Can you work these out from the model? Positions are in its coordinate system, mm. A direction names the side the tool comes from. Give positions to 0.01 mm unless a question says otherwise; leave off trailing zeros. Loops run counter-clockwise (first coordinate to the right, second up) from the corner with the lowest first, then second, coordinate; pieces in that order, holes last. Notation, with made-up numbers: (-19.5, 26) -> (-2.5, 26) arc R27 cw to (-2.5, 43) -> close; hole circle Ø11 at (56, 64). An arc over 180 degrees is marked (long way). Return JSON: item names as keys, results as strings. Group by question number.
Q1. Which directions (+Z, -Z, +X, -X, +Y, -Y) give clear straight access to the entire face, cutting with the end or side of a thin tool? Please do faces 4 (the flat face through (-1.2, -20, -8)), 5 (the cylindrical face through (0.112, -9.86, -5.074)), 6 (the flat face through (0, -36, 0)).
Q2. Suppose I cut it at A-A, the plane z = -8. Please give me the cut outline in (x, y), and give its area (3 significant figures).
Q3. Thinking about a two-plate mould opening in Z: for faces 1 (the flat face through (-4, -20, -8.85)), 2 (the cylindrical face through (-2.947, -27.888, -0.13)), 3 (the flat face through (0.95, -20, -8)), which applies, pulls with the +Z half, pulls with the -Z half, needs draft (parallel to the pull), parting line crosses it, or undercut?
Q4. Will these pins go through, and if not, where does the flat tip stop? pin 1 (4 mm diameter, centred on y = -21, z = 3, fed in from -X); pin 2 (1.7 mm diameter, centred on x = 0, y = -27, fed in from -Z); pin 3 (1 mm diameter, centred on x = 1.5, y = -17.5, fed in from -Z); pin 4 (6 mm diameter, centred on x = 1, y = -28.5, fed in from -Z).
Q5. Suppose I cut it at C-C, the plane y = -12. Please give me the cut outline in (x, z) (3 decimals).
Q6. Suppose I cut it at B-B, the plane x = 0. Please give me the cut outline in (y, z) (3 decimals).
Q7. Suppose I cut it at D-D, the plane z = -2.25. Please give me the cut outline in (x, y).
Q8. I need wall thicknesses on line 1 along Z through (x, y) = (0, -30.5); line 2 along Y through (x, z) = (-2.5, 4.25); line 3 along X through (y, z) = (-21.5, 0.75). Which ranges of each line are inside material? Lowest first, please. Write a range as [from, to].
```python
from build123d import *

# Parameters (mm, degrees)
PAD_DEPTH       = 40
SKETCH001_R     = 5
POCKET_DEPTH    = 20
SKETCH002_R     = 2.95
POCKET001_DEPTH = 16
POCKET002_DEPTH = 40.001
POCKET003_DEPTH = 20


with BuildPart() as part:
    # Sketch → Pad (new body)
    with BuildSketch(Plane.XZ):
        with BuildLine():
            ThreePointArc((5, 0), (0, 5), (-5, 0))
            Line((-5.5, 0), (-5, 0))
            Line((-5.5, -11), (-5.5, 0))
            Line((5.5, -11), (-5.5, -11))
            Line((5.5, 0), (5.5, -11))
            Line((5, 0), (5.5, 0))
        make_face()
    extrude(amount=PAD_DEPTH)

    # Sketch001 (on Face7 of Pad) → Pocket (cut)
    with BuildSketch(Plane(origin=(0, 0, 0), x_dir=(1, 0, 0), z_dir=(0, 1, 0))):
        Circle(SKETCH001_R)
    extrude(amount=-POCKET_DEPTH, mode=Mode.SUBTRACT)

    # Sketch002 (on Face8 of Pocket) → Pocket001 (cut)
    with BuildSketch(Plane(origin=(0, -20, 0), x_dir=(1, 0, 0), z_dir=(0, 1, 0))):
        Circle(SKETCH002_R)
    extrude(amount=-POCKET001_DEPTH, mode=Mode.SUBTRACT)

    # Sketch003 (on Face5 of Pocket001) → Pocket002 (cut, through all)
    with BuildSketch(Plane(origin=(0, 0, 0), x_dir=(1, 0, 0), z_dir=(0, 1, 0))):
        Polygon((-5.5, 11), (3.1, 11), (3.1, 6.7), (0.95, 6.7), (0.95, 8.85), (-1.2, 8.85), (-1.2, 6.7), (-3.35, 6.7), (-3.35, 8.85), (-5.5, 8.85), align=None)
    extrude(amount=-POCKET002_DEPTH, mode=Mode.SUBTRACT)

    # Sketch004 (on Face5 of Pocket002) → Pocket003 (cut)
    with BuildSketch(Plane(origin=(0, 0, 0), x_dir=(1, 0, 0), z_dir=(0, 1, 0))):
        with BuildLine():
            ThreePointArc((5.075, 0), (0, 5.075), (-5.075, 0))
            Line((-5.075, 0), (5.075, 0))
        make_face()
    extrude(amount=-POCKET003_DEPTH, mode=Mode.SUBTRACT)


solid = part.part
```
Ans:
{
 "1": {"face 4": "-Z, +Y, -Y", "face 5": "+Z, +Y", "face 6": "+Y"},
 "2": {"outline": "(-5.5, -40) -> (-3.35, -40) -> (-3.35, 0) -> (-5.5, 0) -> close; (-1.2, -40) -> (0.95, -40) -> (0.95, 0) -> (-1.2, 0) -> close; (3.1, -40) -> (5.5, -40) -> (5.5, 0) -> (3.1, 0) -> close", "area": "268 mm^2"},
 "3": {"face 1": "pulls with the -Z half", "face 2": "undercut", "face 3": "needs draft"},
 "4": {"pin 1": "stops at x = -4.9", "pin 2": "stops at z = -8.85", "pin 3": "stops at z = -6.7", "pin 4": "stops at z = -11"},
 "5": {"outline": "(-5.5, -8.85) -> (-3.35, -8.85) -> (-3.35, -6.7) -> (-1.2, -6.7) -> (-1.2, -8.85) -> (0.95, -8.85) -> (0.95, -6.7) -> (3.1, -6.7) -> (3.1, -11) -> (5.5, -11) -> (5.5, 0) -> (5.075, 0) arc R5.075 cw to (-5.075, 0) -> (-5.5, 0) -> close"},
 "6": {"outline": "(-40, -8.85) -> (0, -8.85) -> (0, -5.075) -> (-20, -5.075) -> (-20, -2.95) -> (-36, -2.95) -> (-36, 2.95) -> (-20, 2.95) -> (-20, 5) -> (-40, 5) -> close"},
 "7": {"outline": "(-5.5, -40) -> (5.5, -40) -> (5.5, 0) -> (4.55, 0) -> (4.55, -20) -> (1.91, -20) -> (1.91, -36) -> (-1.91, -36) -> (-1.91, -20) -> (-4.55, -20) -> (-4.55, 0) -> (-5.5, 0) -> close"},
 "8": {"line 1": "z = [-8.85, -2.95], [2.95, 5]", "line 2": "y = [-40, -20]", "line 3": "x = [-4.94, -2.85], [2.85, 4.94]"}
}
